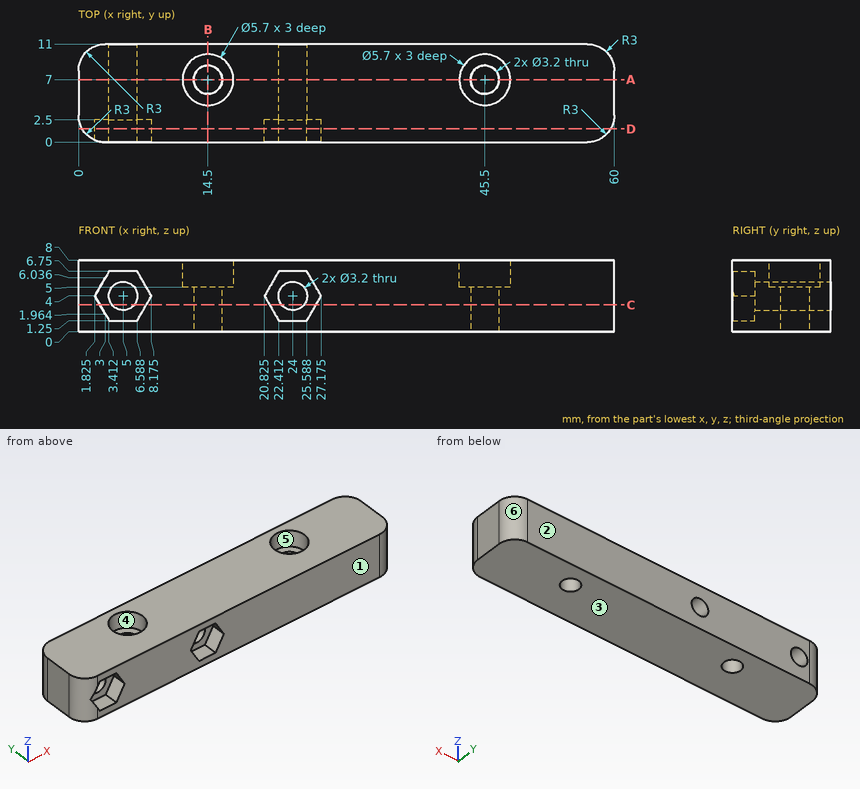
Geometry check sheet. Reference: drawing and pictorial views, mm from the part's lowest x, y, z. A direction names the side the tool comes from. Round coordinates to 2 decimals unless told otherwise and drop trailing zeros. Write each loop counter-clockwise with the first axis right and the second up, starting at its lowest first coordinate (ties: lowest second). Pieces come first, ordered by that corner, then holes.
(1) Section check A-A (y = 7). Enter the section's corners in (x, z).
Returned:
outline: (0, 0) - (12.9, 0) - (12.9, 5) - (11.65, 5) - (11.65, 8) - (0, 8) - close; (16.1, 0) - (43.9, 0) - (43.9, 5) - (42.65, 5) - (42.65, 8) - (17.35, 8) - (17.35, 5) - (16.1, 5) - close; (47.1, 0) - (60, 0) - (60, 8) - (48.35, 8) - (48.35, 5) - (47.1, 5) - close; hole circle Ø3.2 at (5, 4); hole circle Ø3.2 at (24, 4)
(2) Section check B-B (x = 14.5). Enter the section's corners in (y, z), plus the area to 3 significant figures.
Returned:
outline: (0, 0) - (5.4, 0) - (5.4, 5) - (4.15, 5) - (4.15, 8) - (0, 8) - close; (8.6, 0) - (11, 0) - (11, 8) - (9.85, 8) - (9.85, 5) - (8.6, 5) - close
area: 54.9 mm2
(3) Access from +Z, -Z, +X, -X, +Y, -Y to the whole of each face (thin tool, end or side, straight path). Record for the marked faces 5 and 6.
Returned:
face 5: +Z
face 6: +Z, -Z, +X, +Y
(4) Material ranges on line 1 (Z direction, x = 5, y = 4.75); line 2 (X direction, y = 7.75, z = 6.5); line 3 (Y direction, x = 14.5, z = 6.9), recorded low to high.
Returned:
line 1: z = 0 to 2.4, 5.6 to 8
line 2: x = 0 to 11.75, 17.25 to 42.75, 48.25 to 60
line 3: y = 0 to 4.15, 9.85 to 11
(5) Section check C-C (z = 3). Enter the section's corners in (x, y), plus the area to 3 significant figures.
Returned:
outline: (0, 3) arc R3 ccw to (2.4, 0.06) - (2.4, 2.5) - (3.75, 2.5) - (3.75, 11) - (3, 11) arc R3 ccw to (0, 8) - close; (6.25, 2.5) - (7.6, 2.5) - (7.6, 0) - (21.4, 0) - (21.4, 2.5) - (22.75, 2.5) - (22.75, 11) - (6.25, 11) - close; (25.25, 2.5) - (26.6, 2.5) - (26.6, 0) - (57, 0) arc R3 ccw to (60, 3) - (60, 8) arc R3 ccw to (57, 11) - (25.25, 11) - close; hole circle Ø3.2 at (14.5, 7); hole circle Ø3.2 at (45.5, 7)
area: 568 mm2
(6) Mould release check, pull along Y, two halves, no side actions. Record for the marked faces 1, 2, 3 and 4: pulls with the +Y half, pulls with the -Y half, needs draft (parallel to the pull), parting line crosses it, or undercut.
Returned:
face 1: pulls with the -Y half
face 2: pulls with the +Y half
face 3: needs draft
face 4: undercut
(7) Depth check by flat-ended pin: pin 1 Ø1.9 at (x, y) = (45.5, 7) entering from +Z; pin 2 Ø1.6 at (x, z) = (6.5, 3) entering from -Y. Enter the tip coordinate at first touch or a pass-through.
Returned:
pin 1: passes through
pin 2: stops at y = 2.5
(8) Section check D-D (y = 1.5). Give the number of separate pieces and of enclosed holes in the cut face, plus the area to 3 significant figures.
Returned:
separate pieces: 1
enclosed holes: 2
area: 421 mm2
